Could you check a few things on this model? Use its own coordinates, in mm. Face numbers are marked on the shaded views. A direction names the side the tool comes from. Round coordinates to 2 decimals unless told otherwise and drop trailing zeros. Loops run counter-clockwise (first coordinate to the right, second up) from the corner with the lowest first, then second, coordinate; pieces in that order, holes last. Notation, with made-up numbers: (59, 39) -> (99, 39) arc R16 cw to (99, 56) -> close; hole circle Ø4 at (10, -20). An arc over 180 degrees is marked (long way). One line per item, written item: value.
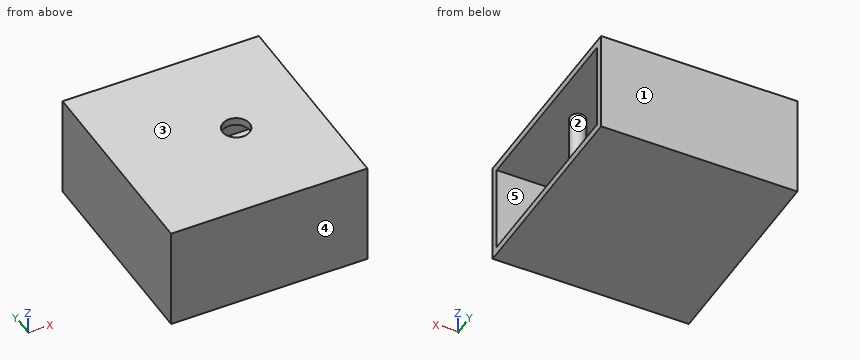
```python
from build123d import *

# Parameters (mm, degrees)
SKETCH_1_W          = 27
SKETCH_1_H          = 54
SKETCH_1_W_2        = 23
SKETCH_1_H_2        = 50
EXTRUDE_1_DEPTH     = 50
SKETCH_2_R          = 3.5
CUT_EXTRUDE_1_DEPTH = 5
SKETCH_3_R          = 2
EXTRUDE_2_DEPTH     = 25
SKETCH_4_W          = 27
SKETCH_4_H          = 54
EXTRUDE_3_DEPTH     = 1


with BuildPart() as part:
    # 草图1 → 凸台-拉伸1 (new body)
    with BuildSketch(Plane(origin=(0, 0, 0), x_dir=(0, 0, -1), z_dir=(1, 0, 0))):
        Rectangle(SKETCH_1_W, SKETCH_1_H)
        Rectangle(SKETCH_1_W_2, SKETCH_1_H_2, mode=Mode.SUBTRACT)
    extrude(amount=EXTRUDE_1_DEPTH)

    # 草图2 → 切除-拉伸1 (cut)
    with BuildSketch(Plane.XY.offset(13.5)):
        with Locations((30, 0)):
            Circle(SKETCH_2_R)
    extrude(amount=-CUT_EXTRUDE_1_DEPTH, mode=Mode.SUBTRACT)

    # 草图3 → 凸台-拉伸2 (add)
    with BuildSketch(Plane.XY.offset(13.5)):
        with Locations((42, 0)):
            Circle(SKETCH_3_R)
    extrude(amount=-EXTRUDE_2_DEPTH)

    # 草图4 → 凸台-拉伸3 (add)
    with BuildSketch(Plane.ZY):
        Rectangle(SKETCH_4_W, SKETCH_4_H)
    extrude(amount=EXTRUDE_3_DEPTH)


solid = part.part
```
Item 1: For the marked faces 4 and 5, which set-ups out of +Z, -Z, +X, -X, +Y, -Y let a thin tool reach every point of the face, with its end or its side?
Output:
face 4: +Z, -Z, +X, -X, -Y
face 5: +X
Item 2: If we mould it in two halves opening along Y, with no side actions, what happens to the marked faces 1, 2 and 3? For each: released by +Y, released by -Y, zero draft, split by the parting line, or undercut.
Output:
face 1: released by +Y
face 2: undercut
face 3: zero draft
Item 3: If we section it at C-C on y = 0: List the corners of the cut face in (x, z) for me, plus the area to 3 significant figures.
Output:
outline: (-1, -13.5) -> (50, -13.5) -> (50, -11.5) -> (44, -11.5) -> (44, 11.5) -> (50, 11.5) -> (50, 13.5) -> (33.5, 13.5) -> (33.5, 11.5) -> (40, 11.5) -> (40, -11.5) -> (0, -11.5) -> (0, 11.5) -> (26.5, 11.5) -> (26.5, 13.5) -> (-1, 13.5) -> close
area: 305 mm²
Item 4: If we section it at A-A on x = 42: List the corners of the cut face in (y, z) for me, plus the area to 3 significant figures.
Output:
outline: (-27, -13.5) -> (27, -13.5) -> (27, 13.5) -> (-27, 13.5) -> close; hole (-25, -11.5) -> (-2, -11.5) -> (-2, 11.5) -> (-25, 11.5) -> close; hole (2, -11.5) -> (25, -11.5) -> (25, 11.5) -> (2, 11.5) -> close
area: 400 mm²
Item 5: I need wall thicknesses on line 1 (Y direction, x = 11.5, z = 5.25); line 2 (Z direction, x = 7.5, y = 24.5); line 3 (Y direction, x = 30, z = 12.5). Which ranges of each line are inside material? Lowest first, please. Write a range as from..to.
Output:
line 1: y = -27..-25, 25..27
line 2: z = -13.5..-11.5, 11.5..13.5
line 3: y = -27..-3.5, 3.5..27
Item 6: If we section it at D-D on x = 30: List the corners of the cut face in (y, z) for me, plus the area to 3 significant figures.
Output:
outline: (-27, -13.5) -> (27, -13.5) -> (27, 13.5) -> (3.5, 13.5) -> (3.5, 11.5) -> (25, 11.5) -> (25, -11.5) -> (-25, -11.5) -> (-25, 11.5) -> (-3.5, 11.5) -> (-3.5, 13.5) -> (-27, 13.5) -> close
area: 294 mm²
Item 7: Will these pins go through, and if not, where does the flat tip stop? pin 1 Ø12 at (y, z) = (12, -3.5) entering from +X; pin 2 Ø6.5 at (x, y) = (30, 0) entering from +Z.
Output:
pin 1: stops at x = 0
pin 2: stops at z = -11.5
Item 8: If we section it at B-B on z = 9.25: List the corners of the cut face in (x, y) for me.
Output:
outline: (-1, -27) -> (50, -27) -> (50, -25) -> (0, -25) -> (0, 25) -> (50, 25) -> (50, 27) -> (-1, 27) -> close; circle Ø4 at (42, 0)
